Here's how the part is built. I have some questions about the finished solid (model axes, mm). Face numbers are marked on the shaded views. A direction names the side the tool comes from. Round coordinates to 2 decimals unless told otherwise and drop trailing zeros. Loops run counter-clockwise (first coordinate to the right, second up) from the corner with the lowest first, then second, coordinate; pieces in that order, holes last. Notation, with made-up numbers: (75, -19) - (106, -19) arc R15 cw to (106, -8) - close; hole circle Ø10 at (21, 87.5). An arc over 180 degrees is marked (long way). Answer as a JSON object with one key per item and string values. Group by question number.
1) I want a section at A-A, the plane z = 0. Please give me the cut outline in (x, y).
2) Will these pins go through, and if not, where does the flat tip stop? P1, Ø2, axis at y = 10, z = -45.5, coming from the -X side; P2, Ø2, axis at x = 5, z = 17, coming from the -Y side; P3, Ø5, axis at x = 24, z = -8.5, coming from the +Y side; P4, Ø22.5, axis at y = 0, z = 0, coming from the -X side.
3) If we mould it in two halves opening along X, with no side actions, what happens to the marked faces 4, 5, 6 and 7? For each: pulls with the +X half, pulls with the -X half, needs draft (parallel to the pull), parting line crosses it, or undercut.
4) I want a section at D-D, the plane x = 33.5. Please give me the cut outline in (y, z), then the cut area to 3 significant figures.
5) Which directions (+Z, -Z, +X, -X, +Y, -Y) give clear straight access to the entire face, cutting with the end or side of a thin tool? Please do the marked faces 1, 2 and 3.
6) I want a section at C-C, the plane x = 1.5. Please give me the cut outline in (y, z).
7) If I drill on line 1 along Y through (x, z) = (-2, 0); line 2 along Z through (x, y) = (27.5, 0); line 3 along X through (y, z) = (-4.5, -23.5), over which ranges is the centre line in solid material (lowest first)? Write a range as [from, to].
Autodesk Inventor part; units mm, degrees
ref_plane "YZ Plane" through (0, 0, 0) normal (1, 0, 0) x (0, 1, 0)
ref_plane "XZ Plane" through (0, 0, 0) normal (0, 1, 0) x (-1, 0, 0)
ref_plane "XY Plane" through (0, 0, 0) normal (0, 0, 1) x (1, 0, 0)
sketch "Sketch1" plane through (0, 0, 0) normal (1, 0, 0) x (0, 1, 0)
  circle A0 centre (0, 0) radius 60
  dimension "d0" = 120
extrude "Extrusion1" add sketch "Sketch1" along normal blind 28
sketch "Sketch2" plane through (28, 0, 0) normal (1, 0, 0) x (0, 0, -1)
  circle A0 centre (0, 0) radius 7
  dimension "d3" = 14
extrude "Extrusion2" cut sketch "Sketch2" against normal blind 28
sketch "Sketch3" plane through (0, 0, 0) normal (0, 1, 0) x (-1, 0, 0)
  line L0 (0, 60) -> (-28, 60)
  line L1 (-4.9193, 60) -> (-9.3746, 44.6454)
  line L2 (-9.3746, 44.6454) -> (-17.9139, 44.6454)
  line L3 (-17.9139, 44.6454) -> (-23.6686, 60)
  line L4 (-4.9193, 60) -> (-23.6686, 60)
  line L5 (-62.3987, 0) -> (62.1852, 0)
  point P0 (0, 0)
revolve "Revolution1" cut sketch "Sketch3" angle 360 about axis through (62.3987, 0, 0) along (-1, 0, 0)
sketch "Sketch4" plane through (28, 0, 0) normal (1, 0, 0) x (0, 0, -1)
  circle A0 centre (0, 0) radius 15
  circle A1 centre (0, 0) radius 7
  dimension "d7" = 30
  dimension "d8" = 14
extrude "Extrusion3" add sketch "Sketch4" along normal blind 11
sketch "Sketch5" plane through (0, 0, 0) normal (-1, 0, 0) x (0, 0, 1)
  circle A0 centre (0, 0) radius 7
  circle A1 centre (0, 0) radius 15
  dimension "d11" = 30
  dimension "d12" = 14
extrude "Extrusion4" add sketch "Sketch5" along normal blind 11
properties part number "Rueda"
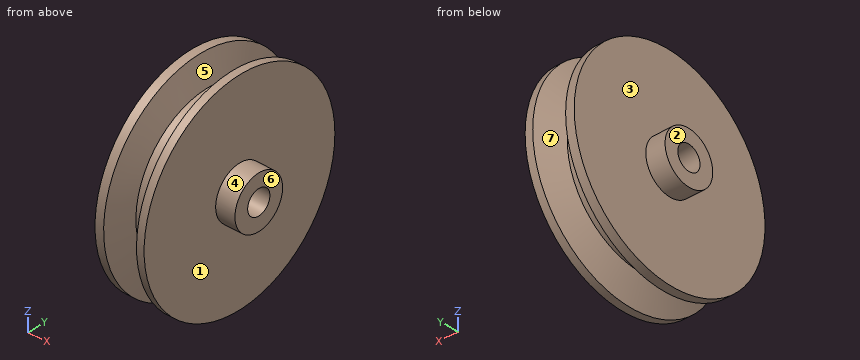
Outcome:
{
 "1": {"outline": "(-11, -15) - (0, -15) - (0, -60) - (4.92, -60) - (9.37, -44.65) - (17.91, -44.65) - (23.67, -60) - (28, -60) - (28, -15) - (39, -15) - (39, -7) - (-11, -7) - close; (-11, 7) - (39, 7) - (39, 15) - (28, 15) - (28, 60) - (23.67, 60) - (17.91, 44.65) - (9.37, 44.65) - (4.92, 60) - (0, 60) - (0, 15) - (-11, 15) - close"},
 "2": {"P1": "x = 0", "P2": "y = -57.83", "P3": "y = 59.7", "P4": "x = -11"},
 "3": {"face 4": "needs draft", "face 5": "undercut", "face 6": "pulls with the +X half", "face 7": "undercut"},
 "4": {"outline": "circle Ø30 at (0, 0); hole circle Ø14 at (0, 0)", "area": "553 mm^2"},
 "5": {"face 1": "+X", "face 2": "+Z, -Z, -X, +Y, -Y", "face 3": "-X"},
 "6": {"outline": "circle Ø120 at (0, 0); hole circle Ø14 at (0, 0)"},
 "7": {"line 1": "[-15, -7], [7, 15]", "line 2": "[-60, -7], [7, 60]", "line 3": "[0, 28]"}
}
